Design review of the part built by this model. Coordinates are the model's own, in mm. A direction names the side the tool comes from. Give positions to 0.01 mm unless a question says otherwise; leave off trailing zeros. Order: outer loops, then holes, each group sorted by start corner. A loop starts at its lowest first (then second) coordinate and runs counter-clockwise, first axis right, second up. Notation, with made-up numbers: (-19, 59.25) -> (31, 59.25) arc R12 ccw to (31, 72.25) -> close; hole circle Ø10 at (-21, -36). An arc over 180 degrees is marked (long way). Return JSON: item names as keys, results as strings.
Autodesk Inventor part; units mm, degrees
ref_plane "YZ Plane" through (0, 0, 0) normal (1, 0, 0) x (0, 1, 0)
ref_plane "XZ Plane" through (0, 0, 0) normal (0, 1, 0) x (-1, 0, 0)
ref_plane "XY Plane" through (0, 0, 0) normal (0, 0, 1) x (1, 0, 0)
sketch "Sketch1" plane through (0, 0, 0) normal (0, 1, 0) x (-1, 0, 0)
  line L0 (210.6, 131) -> (0, 131)
  line L1 (0, 131) -> (0, 0)
  line L2 (0, 0) -> (210.6, 0)
  line L3 (210.6, 0) -> (210.6, 131)
  line L4 (92, 68) -> (7, 68) construction
  line L5 (7, 68) -> (7, 124) construction
  line L6 (7, 124) -> (92, 124) construction
  line L7 (92, 124) -> (92, 68) construction
  circle A0 centre (88.5, 71.5) radius 1.1
  circle A1 centre (88.5, 120.5) radius 1.1
  circle A2 centre (30.5, 71.5) radius 1.1
  circle A3 centre (30.5, 120.5) radius 1.1
  line L8 (0, 0) -> (-136.9444, 0) construction
  line L9 (0, 0) -> (0, -49.9102) construction
  circle A4 centre (88.5, 71.5) radius 2.1
  circle A5 centre (88.5, 120.5) radius 2.1
  circle A6 centre (30.5, 71.5) radius 2.1
  circle A7 centre (30.5, 120.5) radius 2.1
  line L10 (205.6, 66) -> (5, 66)
  line L11 (5, 66) -> (5, 126)
  line L12 (5, 126) -> (205.6, 126)
  line L13 (205.6, 126) -> (205.6, 66)
  line L14 (203.6, 69.33) -> (102, 69.33) construction
  line L15 (102, 69.33) -> (102, 122.67) construction
  line L16 (102, 122.67) -> (203.6, 122.67) construction
  line L17 (203.6, 122.67) -> (203.6, 69.33) construction
  line L18 (205.6, 5) -> (38.6, 5)
  line L19 (38.6, 5) -> (38.6, 63)
  line L20 (38.6, 63) -> (205.6, 63)
  line L21 (205.6, 63) -> (205.6, 5)
  circle A8 centre (188.36, 71.87) radius 2.55
  circle A9 centre (188.36, 71.87) radius 1.55
  circle A10 centre (113.43, 71.87) radius 2.55
  circle A11 centre (113.43, 71.87) radius 1.55
  circle A12 centre (189.63, 120.13) radius 1.55
  circle A13 centre (107.08, 120.13) radius 2.55
  circle A14 centre (189.63, 120.13) radius 2.55
  circle A15 centre (107.08, 120.13) radius 1.55
  circle A16 centre (137.56, 115.05) radius 2.55
  circle A17 centre (137.56, 115.05) radius 1.55
  circle A18 centre (137.56, 87.11) radius 2.55
  circle A19 centre (137.56, 87.11) radius 1.55
  point P0 (92, 96)
  point P1 (102, 96)
  point P2 (1.5544, 63)
  point P3 (2.0056, 63)
  point P4 (82.8344, 63)
  point P5 (83.2856, 63)
  dimension "d8" = 85
  dimension "d9" = 56
  dimension "d10" = 2.2
  dimension "d11" = 3.5
  dimension "d12" = 3.5
  dimension "d13" = 3.5
  dimension "d33" = 1
  dimension "d34" = 1
  dimension "d35" = 1
  dimension "d36" = 1
  dimension "d44" = 58
  dimension "d48" = 53.34
  dimension "d49" = 101.6
  dimension "d50" = 167
  dimension "d51" = 58
  dimension "d52" = 5
  dimension "d55" = 2
  dimension "d56" = 2
  dimension "d57" = 2
  dimension "d58" = 10
  dimension "d59" = 5
  dimension "d60" = 15.24
  dimension "d61" = 2.54
  dimension "d62" = 3.1
  dimension "d63" = 1
  dimension "d64" = 90.17
  dimension "d65" = 13.97
  dimension "d66" = 96.52
  dimension "d68" = 66.04
  dimension "d70" = 45.72
  dimension "d71" = 17.78
  dimension "d73" = 5
  dimension "d74" = 50.8
  dimension "d76" = 3
  dimension "d77" = 2
  dimension "d78" = 5
extrude "Extrusion1" add sketch "Sketch1" against normal blind 2 contours L3 L2 L1 L0 | A0 | A1 | A2 | A3 | A4 | A5 | A6 | A7 | L10 L11 L12 L13 | L18 L19 L20 L21 | A8 | A9 | A10 | A11 | A12 | A13 | A14 | A15 | A16 | A17 | A18 | A19
extrude "Extrusion2" add sketch "Sketch1" along normal blind 5 contours L3 L2 L1 L0
extrude "Extrusion3" add sketch "Sketch1" along normal blind 3 contours A4 | A5 | A6 | A7 | A8 | A10 | A13 | A14 | A16 | A18
fillet "Fillet1" radius 5 4 edges at (-210.6, 1.5, 0) (0, 1.5, 131) (-210.6, 1.5, 131) (0, 1.5, 0)
chamfer "Chamfer1" distance 2 angle 45 8 edges at (-105.3, -2, 131) (-209.1355, -2, 129.5355) (-210.6, -2, 65.5) (-209.1355, -2, 1.4645) (-105.3, -2, 0) (-1.4645, -2, 1.4645) (0, -2, 65.5) (-1.4645, -2, 129.5355)
equation "\"d12\" = d11"
equation "\"d13\" = d11"
equation "\"board_border\" = 2"
equation "\"base_wall\" = 5"
properties part number "Electronic Base"
Item 1: Add section D-D (z = 11.5). Give the boundary of the cut face in (x, y), plus the area to 3 significant figures.
Result set:
{"outline": "(-210.6, 0) -> (-208.6, -2) -> (-2, -2) -> (0, 0) -> (0, 5) -> (-38.6, 5) -> (-38.6, 0) -> (-205.6, 0) -> (-205.6, 5) -> (-210.6, 5) -> close", "area": "635 mm^2"}
Item 2: Machinability: for faces 4 (the face through (-139.916, 1.479, 116.027)), 5 (the face through (-2, 2, 1)), which of the approach directions +Z, -Z, +X, -X, +Y, -Y give a long, thin tool a straight path to every point of the face, cutting with its end or side? Answer none if there is none.
Result set:
{"face 4": "+Y", "face 5": "-Z, +X, +Y, -Y"}
Item 3: Add section B-B (x = -133). Give the boundary of the cut face in (y, z), plus the area to 3 significant figures.
Result set:
{"outline": "(-2, 2) -> (0, 0) -> (5, 0) -> (5, 5) -> (0, 5) -> (0, 63) -> (5, 63) -> (5, 66) -> (0, 66) -> (0, 126) -> (5, 126) -> (5, 131) -> (0, 131) -> (-2, 129) -> close", "area": "323 mm^2"}
Item 4: For pin 1 (2.5 mm diameter, centred on x = -137.5, z = 87, fed in from +Y); pin 2 (2 mm diameter, centred on x = -88, z = 120.5, fed in from +Y), all flat-tipped, find the tip position at first contact; note any pin that passes through.
Result set:
{"pin 1": "stops at y = 0", "pin 2": "stops at y = 3"}
Item 5: Add section C-C (y = 1.25). Give the number of separate pieces and of enclosed holes in the cut face, plus the area to 3 significant figures.
Result set:
{"separate pieces": "11", "enclosed holes": "12", "area": "5,960 mm^2"}
Item 6: Add section A-A (z = 94). Give the boundary of the cut face in (x, y), plus the area to 3 significant figures.
Result set:
{"outline": "(-210.6, 0) -> (-208.6, -2) -> (-2, -2) -> (0, 0) -> (0, 5) -> (-5, 5) -> (-5, 0) -> (-205.6, 0) -> (-205.6, 5) -> (-210.6, 5) -> close", "area": "467 mm^2"}
Item 7: Mouldability with a two-part tool opening along X and no side actions: class faces 1 (the face through (-208.25, -1.21, 2.29)), 2 (the face through (-89.4, 3, 70.6)), 3 (the face through (-2.29, -1.21, 2.35)) as released by +X, released by -X, zero draft, split by the parting line, or undercut.
Result set:
{"face 1": "released by -X", "face 2": "undercut", "face 3": "released by +X"}
Item 8: Wall thickness on L1, parallel to Z at x = -195, y = 3.5; L2, parallel to Z at x = -107.08, y = 1.55; L3, parallel to X at y = 2.25, z = 54.5: over which ranges is each line inside the solid? List them lowest first. Write a range as [from, to].
Result set:
{"L1": "z = [0, 5], [63, 66], [126, 131]", "L2": "z = [0, 5], [63, 66], [117.58, 118.58], [121.68, 122.68], [126, 131]", "L3": "x = [-210.6, -205.6], [-38.6, 0]"}
